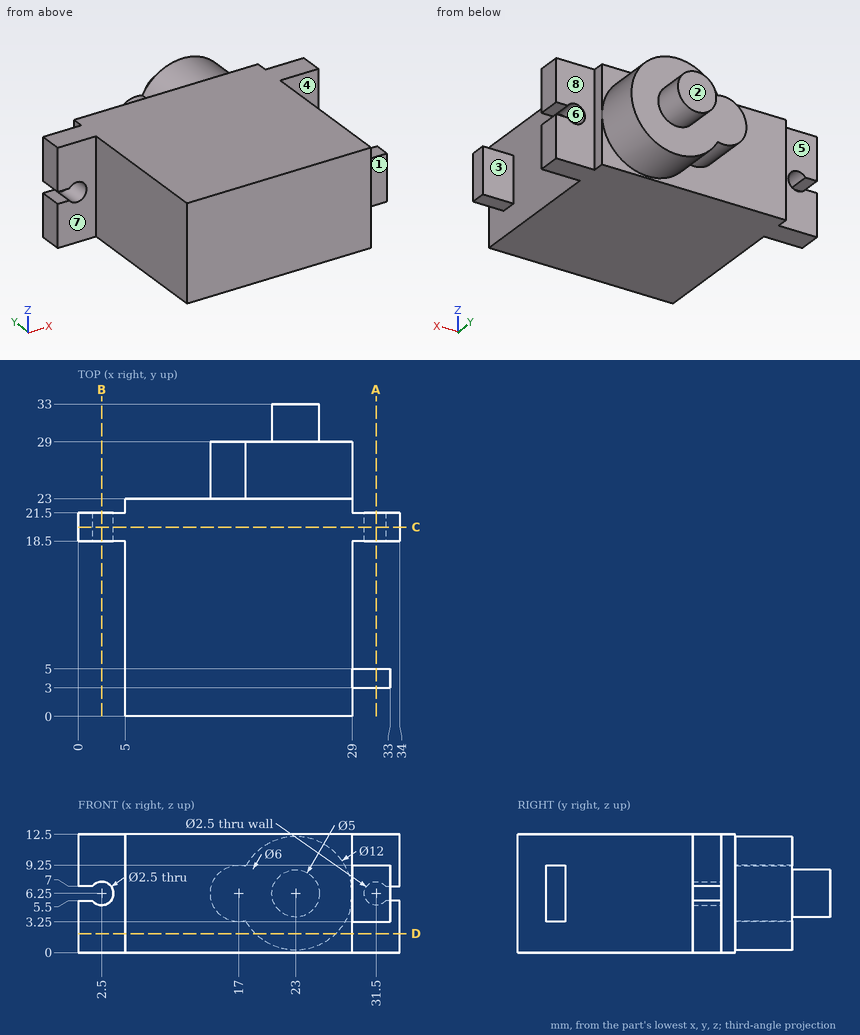
Design review of the part shown in the three views and the two pictorial views. Dimensions are in mm from the part's minimum x, y and z. A direction names the side the tool comes from. Round coordinates to 2 decimals unless told otherwise and drop trailing zeros. Loops run counter-clockwise (first coordinate to the right, second up) from the corner with the lowest first, then second, coordinate; pieces in that order, holes last. Notation, with made-up numbers: (25, 55.25) -> (48, 55.25) arc R12 cw to (48, 59.25) -> close; hole circle Ø7 at (74.25, 75.5). An arc over 180 degrees is marked (long way). Answer as CSV lines item,"result".
1) Draft analysis for pull direction Y (two halves, no side actions). For the marked faces 1, 2 and 3, state which applies: pulls with the +Y half, pulls with the -Y half, needs draft (parallel to the pull), parting line crosses it, or undercut.
Geometry results:
face 1,"pulls with the -Y half"
face 2,"pulls with the +Y half"
face 3,"undercut"
2) Add section A-A on x = 31.5. Write out the cut boundary in (y, z).
Geometry results:
outline,"(3, 3.25) -> (5, 3.25) -> (5, 9.25) -> (3, 9.25) -> close; (18.5, 0) -> (21.5, 0) -> (21.5, 5) -> (18.5, 5) -> close; (18.5, 7.5) -> (21.5, 7.5) -> (21.5, 12.5) -> (18.5, 12.5) -> close"
3) Tool access review of the marked faces 4, 5, 6, 7 and 8: name each direction out of +Z, -Z, +X, -X, +Y, -Y from which nothing blocks a thin tool from reaching the whole face with its end or side.
Geometry results:
face 4,"+Z, -Z, +X"
face 5,"+Z, -Z, -X, +Y"
face 6,"+Y"
face 7,"+Z, -Z, -X, -Y"
face 8,"+Z, -Z, +X, +Y"
4) To check wall thickness, follow line 1 along Z through (x, y) = (2.5, 20.7); line 2 along X through (y, z) = (11.5, 9.5); line 3 along Y through (x, z) = (12.5, 4.5). State the ranges of each line that lie inside material, in increasing order. Write a range as from..to.
Geometry results:
line 1,"z = 0..5, 7.5..12.5"
line 2,"x = 5..29"
line 3,"y = 0..23"
5) For P1, Ø2, axis at y = 4, z = 6, coming from the +X side; P2, Ø5.5, axis at x = 1.5, z = 5.5, coming from the -Y side; P3, Ø2, axis at x = 6, z = 8, coming from the +Y side, all flat-tipped, find the tip position at first contact; note any pin that passes through.
Geometry results:
P1,"stops at x = 33"
P2,"stops at y = 18.5"
P3,"stops at y = 23"
6) Add section B-B on x = 2.5. Write out the cut boundary in (y, z), plus the area to 3 significant figures.
Geometry results:
outline,"(18.5, 0) -> (21.5, 0) -> (21.5, 5) -> (18.5, 5) -> close; (18.5, 7.5) -> (21.5, 7.5) -> (21.5, 12.5) -> (18.5, 12.5) -> close"
area,"30.0 mm²"
7) Add section C-C on y = 20. Write out the cut boundary in (x, z), plus the area to 3 significant figures.
Geometry results:
outline,"(0, 0) -> (34, 0) -> (34, 5.5) -> (32.5, 5.5) arc R1.25 cw (long way) to (32.5, 7) -> (34, 7) -> (34, 12.5) -> (0, 12.5) -> (0, 7) -> (1.5, 7) arc R1.25 cw (long way) to (1.5, 5.5) -> (0, 5.5) -> close"
area,"411 mm²"
8) Add section D-D on z = 2. Write out the cut boundary in (x, y), plus the area to 3 significant figures.
Geometry results:
outline,"(0, 18.5) -> (5, 18.5) -> (5, 0) -> (29, 0) -> (29, 18.5) -> (34, 18.5) -> (34, 21.5) -> (29, 21.5) -> (29, 23) -> (27.24, 23) -> (27.24, 29) -> (18.76, 29) -> (18.76, 23) -> (5, 23) -> (5, 21.5) -> (0, 21.5) -> close"
area,"633 mm²"
